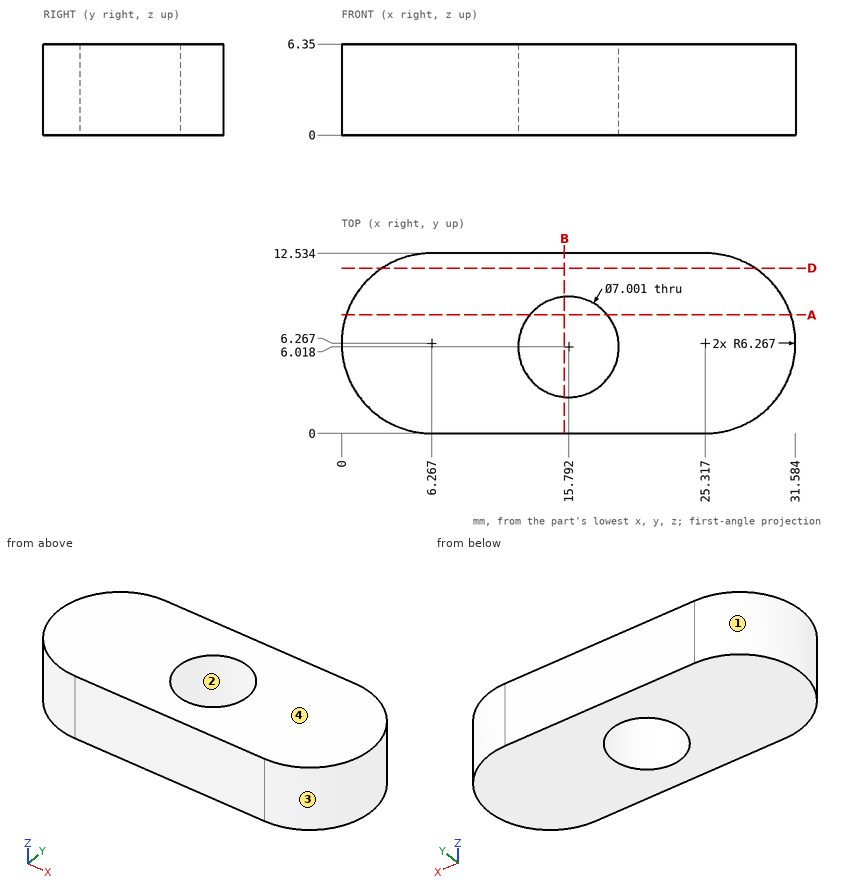
Input: dimensioned drawing with shaded views. Units: mm. Origin: part minimum x, y, z. Give positions to 0.01 mm unless a question says otherwise; leave off trailing zeros. Write each loop counter-clockwise with the first axis right and the second up, starting at its lowest first coordinate (ties: lowest second). Pieces come first, ordered by that corner, then holes. Notation, with made-up numbers: M 37.5,-8.75 L 84.5,-8.75 A35 cw 84.5,28.25 Z; hole C 40,49.25 d10. An arc over 180 degrees is marked long. Return JSON: item names as keys, results as strings. Group by question number.
1) Cut plane D-D, the plane y = 11.5. Output: boundary loops of the cut face in (x, z), plus the area to 3 significant figures.
2) Pin query (flat end, axial travel): P1, Ø3, axis at y = 9.5, z = 3.5, coming from the +X side; P2, Ø3, axis at y = 1.5, z = 1, coming from the -X side; P3, Ø6, axis at x = 12.5, y = 1.5, coming from the -Z side. Return the tip coordinate at first contact, or that it passes through.
3) Cut plane B-B, the plane x = 15.5. Output: boundary loops of the cut face in (y, z), plus the area to 3 significant figures.
4) Pull-direction query (X, two-part tool) for the marked faces 1, 2, 3 and 4; classes: pulls with the +X half, pulls with the -X half, needs draft (parallel to the pull), parting line crosses it, or undercut.
5) Material intervals for line 1 along Y through (x, z) = (14.5, 6.25) (1 decimal); line 2 along X through (y, z) = (4.75, 2) (1 decimal); line 3 along Y through (x, z) = (15.5, 6.25), sorted ascending. Write a range as [from, to].
6) Cut plane A-A, the plane y = 8.25. Output: boundary loops of the cut face in (x, z).
Recorded:
{
 "1": {"outline": "M 2.82,0 L 28.77,0 L 28.77,6.35 L 2.82,6.35 Z", "area": "165 mm²"},
 "2": {"P1": "stops at x = 31.34", "P2": "stops at x = 0.92", "P3": "stops at z = 0"},
 "3": {"outline": "M 0,0 L 2.53,0 L 2.53,6.35 L 0,6.35 Z; M 9.51,0 L 12.53,0 L 12.53,6.35 L 9.51,6.35 Z", "area": "35.3 mm²"},
 "4": {"face 1": "pulls with the -X half", "face 2": "undercut", "face 3": "pulls with the +X half", "face 4": "needs draft"},
 "5": {"line 1": "y = [0, 2.8], [9.3, 12.5]", "line 2": "x = [0.2, 12.5], [19.1, 31.4]", "line 3": "y = [0, 2.53], [9.51, 12.53]"},
 "6": {"outline": "M 0.32,0 L 13.1,0 L 13.1,6.35 L 0.32,6.35 Z; M 18.49,0 L 31.26,0 L 31.26,6.35 L 18.49,6.35 Z"}
}
